from build123d import *

# Parameters (mm, degrees)
F1_W     = 3.807
F1_H     = 2.9409
F1_R     = 0.0629689606
F1_R_2   = 0.0630157123
F1_R_3   = 0.0630453805
F2_DEPTH = 0.063
F3_SCALE = 25.4


with BuildPart() as f2:
    # F1 (on Front) → F2 (new body)
    with BuildSketch(Plane.XZ):
        Rectangle(F1_W, F1_H)
        with Locations((-1.6654, -1.09645)):
            Circle(F1_R, mode=Mode.SUBTRACT)
        with Locations((1.6654, -1.09645)):
            Circle(F1_R_2, mode=Mode.SUBTRACT)
        with Locations((-1.6654, 1.09645)):
            Circle(F1_R_3, mode=Mode.SUBTRACT)
        with Locations((1.6654, 1.09645)):
            Circle(F1_R_2, mode=Mode.SUBTRACT)
    extrude(amount=F2_DEPTH)


with BuildPart() as f2_1:
    # F3: moved
    add(f2.part.scale(F3_SCALE).moved(Location((-46.4454, 1.5372, 35.87898))))


solid = f2_1.part
Can you work these out from the model? Positions are in its coordinate system, mm. Coordinates: 2 decimals unless noted, no trailing zeros. Return JSON: item names as keys, results as strings. Group by question number.
Item 1: Thinking about a two-plate mould opening in X: for faces 1 (the flat face through (-47, -0.063, 36)), 2 (the cylindrical face through (-3.284, 0.748, 65.078)), which applies, released by +X, released by -X, zero draft, split by the parting line, or undercut?
Item 2: I'm going to push flat-ended pins straight in: pin 1 Ø3 at (x, z) = (-88.75, 8.03) entering from +Y; pin 2 Ø5 at (x, z) = (-4.14, 8.03) entering from +Y. Where does each tip first touch, or does it pass through?
Item 3: If I drill on L1, parallel to X at y = 0.1, z = 65, over which ranges is the centre line in solid material (lowest first)? Write a range as from..to.
Verdict:
{
 "1": {"face 1": "zero draft", "face 2": "undercut"},
 "2": {"pin 1": "passes through", "pin 2": "stops at y = 1.54"},
 "3": {"L1": "x = -94.79..-89.72, -87.77..-5.12, -3.17..1.9"}
}
